Verification items for the finished model (mm, model axes). Face numbers are marked on the shaded views. A direction names the side the tool comes from. Give positions to 0.01 mm unless a question says otherwise; leave off trailing zeros. Loops run counter-clockwise (first coordinate to the right, second up) from the corner with the lowest first, then second, coordinate; pieces in that order, holes last. Notation, with made-up numbers: (16, 45.5) - (66, 45.5) arc R23 cw to (66, 77.5) - close; hole circle Ø5 at (21, 23.5). An arc over 180 degrees is marked (long way). Put each result on its own line as item: value. Start each with the question number.
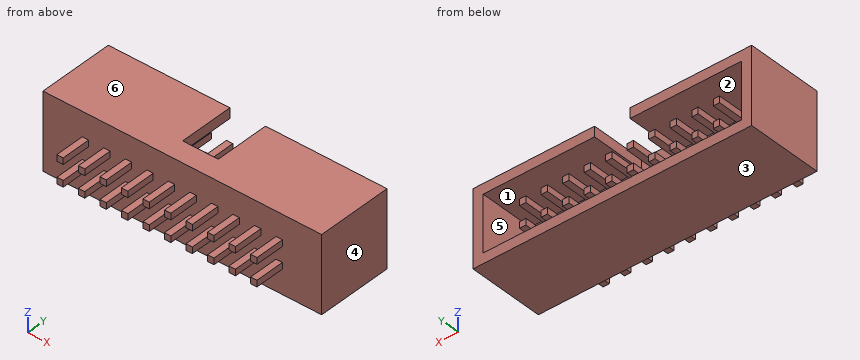
```python
from build123d import *

# Parameters (mm, degrees)
SKETCH_1_W           = 32.88
SKETCH_1_H           = 9
EXTRUDE_1_DEPTH      = 9
SKETCH_2_W           = 30.48
SKETCH_2_H           = 6.6
CUT_EXTRUDE_1_DEPTH  = 6.5
SKETCH_3_W           = 4.2
SKETCH_3_H           = 6.5
CUT_EXTRUDE_2_DEPTH  = 6.5
EXTRUDE_2_DEPTH      = 3.5
EXTRUDE_2_DEPTH_BACK = 8
SKETCH_5_W           = 0.75
SKETCH_5_H           = 0.75


with BuildPart() as part:
    # 草图1 → 拉伸1 (new body)
    with BuildSketch(Plane(origin=(0, 0, 0), x_dir=(1, 0, 0), z_dir=(0, 1, 0))):
        Rectangle(SKETCH_1_W, SKETCH_1_H)
    extrude(amount=EXTRUDE_1_DEPTH)

    # 草图2 → 切除-拉伸1 (cut)
    with BuildSketch(Plane(origin=(0, 9, 0), x_dir=(-1, 0, 0), z_dir=(0, 1, 0))):
        Rectangle(SKETCH_2_W, SKETCH_2_H)
    extrude(amount=-CUT_EXTRUDE_1_DEPTH, mode=Mode.SUBTRACT)

    # 草图3 → 切除-拉伸2 (cut)
    with BuildSketch(Plane.XY.offset(4.5)):
        with Locations((0, 5.75)):
            Rectangle(SKETCH_3_W, SKETCH_3_H)
    extrude(amount=-CUT_EXTRUDE_2_DEPTH, mode=Mode.SUBTRACT)

    # 草图5 → 拉伸2 (add, two sides: drawn at the far end of the back side and taken through both)
    with BuildSketch(Plane.XZ.offset(-EXTRUDE_2_DEPTH_BACK)):
        with Locations((-1.27, 1.27)):
            Rectangle(SKETCH_5_W, SKETCH_5_H)
        with Locations((1.27, 1.27)):
            Rectangle(SKETCH_5_W, SKETCH_5_H)
        with Locations((3.81, 1.27)):
            Rectangle(SKETCH_5_W, SKETCH_5_H)
        with Locations((6.35, 1.27)):
            Rectangle(SKETCH_5_W, SKETCH_5_H)
        with Locations((8.89, 1.27)):
            Rectangle(SKETCH_5_W, SKETCH_5_H)
        with Locations((11.43, 1.27)):
            Rectangle(SKETCH_5_W, SKETCH_5_H)
        with Locations((1.27, -1.27)):
            Rectangle(SKETCH_5_W, SKETCH_5_H)
        with Locations((3.81, -1.27)):
            Rectangle(SKETCH_5_W, SKETCH_5_H)
        with Locations((6.35, -1.27)):
            Rectangle(SKETCH_5_W, SKETCH_5_H)
        with Locations((8.89, -1.27)):
            Rectangle(SKETCH_5_W, SKETCH_5_H)
        with Locations((11.43, -1.27)):
            Rectangle(SKETCH_5_W, SKETCH_5_H)
        with Locations((-3.81, 1.27)):
            Rectangle(SKETCH_5_W, SKETCH_5_H)
        with Locations((-6.35, 1.27)):
            Rectangle(SKETCH_5_W, SKETCH_5_H)
        with Locations((-8.89, 1.27)):
            Rectangle(SKETCH_5_W, SKETCH_5_H)
        with Locations((-11.43, 1.27)):
            Rectangle(SKETCH_5_W, SKETCH_5_H)
        with Locations((-1.27, -1.27)):
            Rectangle(SKETCH_5_W, SKETCH_5_H)
        with Locations((-3.81, -1.27)):
            Rectangle(SKETCH_5_W, SKETCH_5_H)
        with Locations((-6.35, -1.27)):
            Rectangle(SKETCH_5_W, SKETCH_5_H)
        with Locations((-8.89, -1.27)):
            Rectangle(SKETCH_5_W, SKETCH_5_H)
        with Locations((-11.43, -1.27)):
            Rectangle(SKETCH_5_W, SKETCH_5_H)
    extrude(amount=EXTRUDE_2_DEPTH + EXTRUDE_2_DEPTH_BACK)


solid = part.part
```
1) Section check B-B, the plane x = 0.5. Enter the section's corners in (y, z).
2) Draft check along Z on the marked faces 1, 2, 3 and 4. Enter one of: pulls with the +Z half, pulls with the -Z half, needs draft (parallel to the pull), parting line crosses it, or undercut.
3) Set-up check for the marked faces 5 and 6: record each of +Z, -Z, +X, -X, +Y, -Y from which the full face is reachable in a straight line by a thin tool's end or side.
4) Depth check by flat-ended pin: P1, Ø0.8, axis at x = -9, z = -1, coming from the +Y side; P2, Ø4, axis at x = 11, z = -2.5, coming from the -Y side; P3, Ø0.6, axis at y = -1, z = 1, coming from the +X side (3 decimals). Enter the tip coordinate at first touch or a pass-through.
5) Section check A-A, the plane z = 0.25. Enter the section's corners in (x, y).
6) Scan lines: line 1 along Z through (x, y) = (1, 5) (3 decimals); line 2 along Z through (x, y) = (-4, 3) (3 decimals); line 3 along X through (y, z) = (3, 0.5). Record each from-to range of solid material in increasing order. Write a range as from..to.
7) Section check C-C, the plane y = 3.25. State how many separate pieces and enclosed holes the cut face has, plus the area to 3 significant figures.
Results are:
1. outline: (0, -4.5) - (9, -4.5) - (9, -3.3) - (2.5, -3.3) - (2.5, 4.5) - (0, 4.5) - close
2. face 1: undercut
2. face 2: undercut
2. face 3: pulls with the -Z half
2. face 4: needs draft
3. face 5: +Y
3. face 6: +Z, +X, -X, +Y, -Y
4. P1: stops at y = 8
4. P2: stops at y = -3.5
4. P3: stops at x = 11.805
5. outline: (-16.44, 0) - (16.44, 0) - (16.44, 9) - (15.24, 9) - (15.24, 2.5) - (-15.24, 2.5) - (-15.24, 9) - (-16.44, 9) - close
6. line 1: z = -4.5..-3.3, -1.645..-0.895, 0.895..1.645
6. line 2: z = -4.5..-3.3, -1.645..-0.895, 0.895..1.645, 3.3..4.5
6. line 3: x = -16.44..-15.24, 15.24..16.44
7. separate pieces: 21
7. enclosed holes: 0
7. area: 101 mm2
